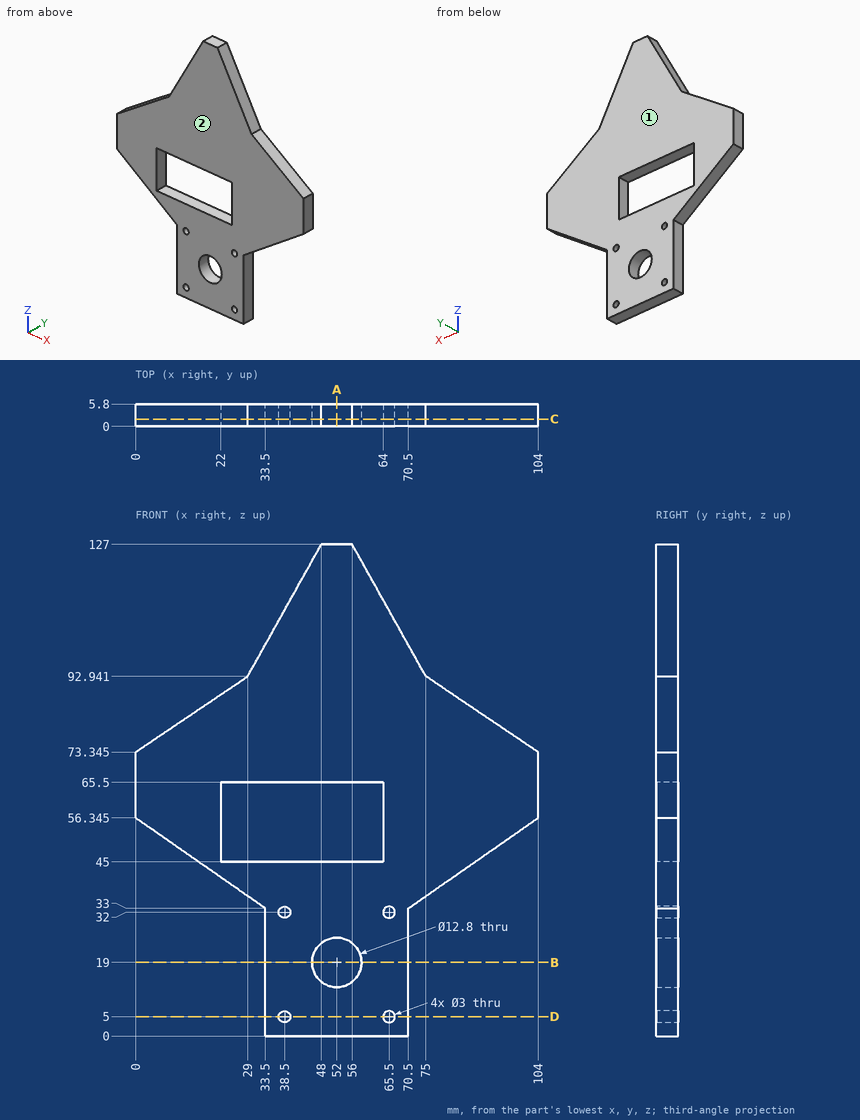
Design review of the part shown in the three views and the two pictorial views. Dimensions are in mm from the part's minimum x, y and z. Round coordinates to 2 decimals unless told otherwise and drop trailing zeros. Write each loop counter-clockwise with the first axis right and the second up, starting at its lowest first coordinate (ties: lowest second). Pieces come first, ordered by that corner, then holes. Notation, with made-up numbers: M 43,87 L 78,87 A20 cw 78,100 Z; hole C 61,84.5 d7. An arc over 180 degrees is marked long. Use a Markdown table: item, result. Add a question column.
Q1. Insertion check: pin 1 (1 mm diameter, centred on y = 4.5, z = 46.5, fed in from +X); pin 2 (3 mm diameter, centred on x = 37, y = 3.5, fed in from +Z); pin 3 (3 mm diameter, centred on y = 2, z = 19.5, fed in from -X). Each pin has a flat end and moves straight along its axis. Give the tip position at first contact, or say it passes through.
Q2. We need section D-D, the plane z = 5. State the section outline as (x, y) points.
Q3. We need section A-A, the plane x = 52. State the section outline as (y, z) points.
Q4. We need section C-C, the plane y = 1.9. State the section outline as (x, z) points (1 decimal), plus the area to 3 significant figures.
Q5. We need section B-B, the plane z = 19. State the section outline as (x, y) points.
Q6. The part is to be moulded in two halves that separate along Y. For the marked faces 1 and 2, say which applies: pulls with the +Y half, pulls with the -Y half, needs draft (parallel to the pull), parting line crosses it, or undercut.
Q7. To check wall thickness, follow line 1 (X direction, y = 4.4, z = 32); line 2 (X direction, y = 2.6, z = 31); line 3 (X direction, y = 3.35, z = 19). State the ranges of each line that lie inside material, in increasing order.
Findings below:
| question | item | result |
|---|---|---|
| 1 | pin 1 | stops at x = 90.59 |
| 1 | pin 2 | stops at z = 109.97 |
| 1 | pin 3 | stops at x = 33.5 |
| 2 | outline | M 33.5,0 L 37,0 L 37,5.8 L 33.5,5.8 Z; M 40,0 L 64,0 L 64,5.8 L 40,5.8 Z; M 67,0 L 70.5,0 L 70.5,5.8 L 67,5.8 Z |
| 3 | outline | M 0,0 L 5.8,0 L 5.8,12.6 L 0,12.6 Z; M 0,25.4 L 5.8,25.4 L 5.8,45 L 0,45 Z; M 0,65.5 L 5.8,65.5 L 5.8,127 L 0,127 Z |
| 4 | outline | M 0,56.3 L 33.5,33 L 33.5,0 L 70.5,0 L 70.5,33 L 104,56.3 L 104,73.3 L 75,92.9 L 56,127 L 48,127 L 29,92.9 L 0,73.3 Z; hole M 22,45 L 64,45 L 64,65.5 L 22,65.5 Z; hole C 38.5,5 d3; hole C 38.5,32 d3; hole C 52,19 d12.8; hole C 65.5,5 d3; hole C 65.5,32 d3 |
| 4 | area | 6,010 mm² |
| 5 | outline | M 33.5,0 L 45.6,0 L 45.6,5.8 L 33.5,5.8 Z; M 58.4,0 L 70.5,0 L 70.5,5.8 L 58.4,5.8 Z |
| 6 | face 1 | pulls with the +Y half |
| 6 | face 2 | pulls with the -Y half |
| 7 | line 1 | x = 33.5 to 37, 40 to 64, 67 to 70.5 |
| 7 | line 2 | x = 33.5 to 37.38, 39.62 to 64.38, 66.62 to 70.5 |
| 7 | line 3 | x = 33.5 to 45.6, 58.4 to 70.5 |
